Input: part model. Units: mm. Frame: model coordinates. A direction names the side the tool comes from. Give positions to 0.01 mm unless a question says otherwise; leave off trailing zeros. Answer as a JSON object with one key per item and string values. Group by question number.
(1) Mould query, pull axis X, two halves, no side actions, for faces 1 (the flat face through (0, 8, -280)), 2 (the cylindrical face through (1.436, 12.386, -196.536)). Classes: +X half, -X half, draft (parallel to the pull), parting line (faces both ways), or undercut.
(2) Section query A-A (x = 0). Count the separate pieces of the cut face and the enclosed holes in it, plus the area to 3 significant figures.
(3) Access query for faces 3 (the flat face through (0.8, 9.7, -142.4)), 4 (the cylindrical face through (0.86, 4.92, -197.92)). Directions: +Z, -Z, +X, -X, +Y, -Y. A direction counts if a zero-diameter tool reaches every point of the face in a straight line with its end or side. Return the directions, or none.
(4) Material intervals for L1, parallel to Z at x = 0.25, y = 9.5; L2, parallel to Z at x = -0.5, y = 11.5; L3, parallel to X at y = 12.25, z = -17, sorted ascending.
(5) Pin query (flat end, axial travel): P1, Ø1.1, axis at y = 8, z = -179, coming from the -X side; P2, Ø6, axis at x = 0, z = -260, coming from the +Y side; P3, Ø1.1, axis at y = 7.5, z = -155, coming from the +X side. Return the tip coordinate at first contact, or that it passes through.
```python
from build123d import *

# Parameters (mm, degrees)
BODY_DEPTH                                 = 280
AESTHETIC_CHAMFER_SIZE                     = 0.15
PRODUCTION_FILLET_R                        = 0.1
MOUNTING_HOLES_PATTERN_COUNT               = 5
MOUNTING_HOLES_PATTERN_PITCH               = 60
PRODUCTION_FILLET_OF_MOUNTING_HOLES_PATT_R = 0.1


with BuildPart() as part:
    # Rail Profile → Body (new body)
    with BuildSketch(Plane.XY):
        with BuildLine():
            Line((-7, 0), (7, 0))
            Line((7, 0), (7.5, 0.5))
            Line((7.5, 0.5), (7.5, 3.085786438))
            ThreePointArc((7.5, 3.085786438), (7.423879533, 3.46846987), (7.207106781, 3.792893219))
            Line((7.207106781, 3.792893219), (4.867157288, 6.132842712))
            ThreePointArc((4.867157288, 6.132842712), (4.780448187, 6.262612052), (4.75, 6.415685425))
            Line((4.75, 6.415685425), (4.75, 8.584314575))
            ThreePointArc((4.75, 8.584314575), (4.780448187, 8.737387948), (4.867157288, 8.867157288))
            Line((4.867157288, 8.867157288), (5.062965362, 9.062965362))
            ThreePointArc((5.062965362, 9.062965362), (5.134996734, 9.161242682), (5.17409812, 9.27664646))
            ThreePointArc((5.17409812, 9.27664646), (5.61862915, 10.13137085), (6.47335354, 10.57590188))
            ThreePointArc((6.47335354, 10.57590188), (6.694124352, 10.694306692), (6.801170165, 10.920803148))
            ThreePointArc((6.801170165, 10.920803148), (6.915305692, 11.154571658), (7.149074202, 11.268707185))
            ThreePointArc((7.149074202, 11.268707185), (7.399691242, 11.400760606), (7.5, 11.665685425))
            Line((7.5, 11.665685425), (7.5, 12.334314575))
            ThreePointArc((7.5, 12.334314575), (7.399691242, 12.599239394), (7.149074202, 12.731292815))
            ThreePointArc((7.149074202, 12.731292815), (6.915305692, 12.845428342), (6.801170165, 13.079196852))
            ThreePointArc((6.801170165, 13.079196852), (6.694124352, 13.305693308), (6.47335354, 13.42409812))
            ThreePointArc((6.47335354, 13.42409812), (5.61862915, 13.86862915), (5.17409812, 14.72335354))
            ThreePointArc((5.17409812, 14.72335354), (5.134996734, 14.838757318), (5.062965362, 14.937034638))
            Line((5.062965362, 14.937034638), (5, 15))
            Line((5, 15), (-5, 15))
            Line((-5, 15), (-5.062965362, 14.937034638))
            ThreePointArc((-5.062965362, 14.937034638), (-5.134996734, 14.838757318), (-5.17409812, 14.72335354))
            ThreePointArc((-5.17409812, 14.72335354), (-5.61862915, 13.86862915), (-6.47335354, 13.42409812))
            ThreePointArc((-6.47335354, 13.42409812), (-6.694124352, 13.305693308), (-6.801170165, 13.079196852))
            ThreePointArc((-6.801170165, 13.079196852), (-6.915305692, 12.845428342), (-7.149074202, 12.731292815))
            ThreePointArc((-7.149074202, 12.731292815), (-7.399691242, 12.599239394), (-7.5, 12.334314575))
            Line((-7.5, 12.334314575), (-7.5, 11.665685425))
            ThreePointArc((-7.5, 11.665685425), (-7.399691242, 11.400760606), (-7.149074202, 11.268707185))
            ThreePointArc((-7.149074202, 11.268707185), (-6.915305692, 11.154571658), (-6.801170165, 10.920803148))
            ThreePointArc((-6.801170165, 10.920803148), (-6.694124352, 10.694306692), (-6.47335354, 10.57590188))
            ThreePointArc((-6.47335354, 10.57590188), (-5.61862915, 10.13137085), (-5.17409812, 9.27664646))
            ThreePointArc((-5.17409812, 9.27664646), (-5.134996734, 9.161242682), (-5.062965362, 9.062965362))
            Line((-5.062965362, 9.062965362), (-4.867157288, 8.867157288))
            ThreePointArc((-4.867157288, 8.867157288), (-4.780448187, 8.737387948), (-4.75, 8.584314575))
            Line((-4.75, 8.584314575), (-4.75, 6.415685425))
            ThreePointArc((-4.75, 6.415685425), (-4.780448187, 6.262612052), (-4.867157288, 6.132842712))
            Line((-4.867157288, 6.132842712), (-7.207106781, 3.792893219))
            ThreePointArc((-7.207106781, 3.792893219), (-7.423879533, 3.46846987), (-7.5, 3.085786438))
            Line((-7.5, 3.085786438), (-7.5, 0.5))
            Line((-7.5, 0.5), (-7, 0))
        make_face()
    extrude(amount=-BODY_DEPTH)

    # Aesthetic Chamfer
    aesthetic_chamfer_edges = [part.edges().sort_by_distance(p)[0] for p in [
        (7.423879533, 3.46846987, -280),
        (-5.134996734, 9.161242682, -280),
        (-4.965061325, 8.965061325, -280),
        (-4.780448187, 8.737387948, -280),
        (-4.75, 7.5, -280),
        (-4.780448187, 6.262612052, -280),
        (-6.037132034, 4.962867966, -280),
        (-7.423879533, 3.46846987, -280),
        (-7.5, 1.792893219, -280),
        (-7.25, 0.25, -280),
        (0, 0, -280),
        (6.037132034, 4.962867966, -280),
        (4.780448187, 6.262612052, -280),
        (4.75, 7.5, -280),
        (4.780448187, 8.737387948, -280),
        (4.965061325, 8.965061325, -280),
        (5.134996734, 9.161242682, -280),
        (5.61862915, 10.13137085, -280),
        (6.694124352, 10.694306692, -280),
        (0, 0, 0),
        (-7.25, 0.25, 0),
        (-7.5, 1.792893219, 0),
        (-7.423879533, 3.46846987, 0),
        (-6.037132034, 4.962867966, 0),
        (-4.780448187, 6.262612052, 0),
        (6.915305692, 11.154571658, -280),
        (-4.75, 7.5, 0),
        (-4.780448187, 8.737387948, 0),
        (-4.965061325, 8.965061325, 0),
        (-5.134996734, 9.161242682, 0),
        (-5.61862915, 10.13137085, 0),
        (-6.694124352, 10.694306692, 0),
        (-6.915305692, 11.154571658, 0),
        (7.25, 0.25, -280),
        (7.399691242, 11.400760606, -280),
        (-7.399691242, 11.400760606, 0),
        (-7.5, 12, 0),
        (-7.399691242, 12.599239394, 0),
        (-6.915305692, 12.845428342, 0),
        (-6.694124352, 13.305693308, 0),
        (-5.61862915, 13.86862915, 0),
        (-5.134996734, 14.838757318, 0),
        (-5.031482681, 14.968517319, 0),
        (7.5, 12, -280),
        (0, 15, 0),
        (5.031482681, 14.968517319, 0),
        (5.134996734, 14.838757318, 0),
        (5.61862915, 13.86862915, 0),
        (6.694124352, 13.305693308, 0),
        (6.915305692, 12.845428342, 0),
        (7.399691242, 12.599239394, 0),
        (7.399691242, 12.599239394, -280),
        (7.5, 12, 0),
        (7.399691242, 11.400760606, 0),
        (6.915305692, 11.154571658, 0),
        (6.694124352, 10.694306692, 0),
        (5.61862915, 10.13137085, 0),
        (5.134996734, 9.161242682, 0),
        (4.965061325, 8.965061325, 0),
        (4.780448187, 8.737387948, 0),
        (6.915305692, 12.845428342, -280),
        (4.75, 7.5, 0),
        (4.780448187, 6.262612052, 0),
        (6.037132034, 4.962867966, 0),
        (7.423879533, 3.46846987, 0),
        (7.5, 1.792893219, 0),
        (7.25, 0.25, 0),
        (6.694124352, 13.305693308, -280),
        (5.61862915, 13.86862915, -280),
        (5.134996734, 14.838757318, -280),
        (5.031482681, 14.968517319, -280),
        (0, 15, -280),
        (-5.031482681, 14.968517319, -280),
        (7.5, 1.792893219, -280),
        (-5.134996734, 14.838757318, -280),
        (-5.61862915, 13.86862915, -280),
        (-6.694124352, 13.305693308, -280),
        (-6.915305692, 12.845428342, -280),
        (-7.399691242, 12.599239394, -280),
        (-7.5, 12, -280),
        (-7.399691242, 11.400760606, -280),
        (-6.915305692, 11.154571658, -280),
        (-6.694124352, 10.694306692, -280),
        (-5.61862915, 10.13137085, -280),
    ]]
    chamfer(aesthetic_chamfer_edges, length=AESTHETIC_CHAMFER_SIZE)

    # Sketch1 → Mounting Hole (revolve, cut)
    with BuildSketch(Plane(origin=(0, 15, -20), x_dir=(0, 0, 1), z_dir=(1, 0, 0))):
        Polygon((0, 0), (0, 15), (2.35, 15), (2.25, 14.9), (2.25, 5.4), (2.35, 5.3), (3.75, 5.3), (3.75, 0.1), (3.85, 0), align=None)
    mounting_hole = revolve(axis=Axis((0, 21.35, -20), (0, -1, 0)), mode=Mode.SUBTRACT)

    # Production Fillet
    production_fillet_edges = [part.edges().sort_by_distance(p)[0] for p in [
        (0, 9.7, -23.75),
    ]]
    fillet(production_fillet_edges, radius=PRODUCTION_FILLET_R)

    # Mounting Holes Pattern: Mounting Hole ×5
    with Locations(*[(0, 0, -i * MOUNTING_HOLES_PATTERN_PITCH) for i in range(1, MOUNTING_HOLES_PATTERN_COUNT)]):
        add(mounting_hole, mode=Mode.SUBTRACT)

    # Production Fillet of Mounting Holes Patt
    production_fillet_of_mounting_holes_patt_edges = [part.edges().sort_by_distance(p)[0] for p in [
        (0, 9.7, -83.75),
        (0, 9.7, -143.75),
        (0, 9.7, -203.75),
        (0, 9.7, -263.75),
    ]]
    fillet(production_fillet_of_mounting_holes_patt_edges, radius=PRODUCTION_FILLET_OF_MOUNTING_HOLES_PATT_R)


solid = part.part
```
Recorded:
{
 "1": {"face 1": "draft", "face 2": "undercut"},
 "2": {"separate pieces": "6", "enclosed holes": "0", "area": "3,780 mm^2"},
 "3": {"face 3": "+Y", "face 4": "+Y, -Y"},
 "4": {"L1": "z = -280 to -262.24, -257.76 to -202.24, -197.76 to -142.24, -137.76 to -82.24, -77.76 to -22.24, -17.76 to 0", "L2": "z = -280 to -263.72, -256.28 to -203.72, -196.28 to -143.72, -136.28 to -83.72, -76.28 to -23.72, -16.28 to 0", "L3": "x = -7.5 to -2.25, 2.25 to 7.5"},
 "5": {"P1": "stops at x = -4.75", "P2": "stops at y = 9.7", "P3": "stops at x = 4.75"}
}
